Verification items for this drawing (mm, ordinates from the low corner). Round coordinates to 2 decimals unless told otherwise and drop trailing zeros. Order: outer loops, then holes, each group sorted by start corner. A loop starts at its lowest first (then second) coordinate and runs counter-clockwise, first axis right, second up. Notation, with made-up numbers: (31, -6.75) - (43, -6.75) arc R29 cw to (43, 21.25) - close; hole circle Ø11 at (-14.75, -1). An arc over 180 degrees is marked (long way). Use a Markdown table: item, result. Add a question column.
(1) Thickness scan on line 1 along Z through (x, y) = (49, 15); line 2 along Z through (x, y) = (30, 8) (1 decimal); line 3 along X through (y, z) = (27.5, 47.5) (1 decimal). Record the ranges inside material, lowest first. Write a range as [from, to].
(2) Section check A-A on y = 8. Record the boundary of the cut face in (x, z), then the cut area to 3 significant figures.
(3) Gauge pin test, flat ends, axial feed: P1, Ø5, axis at x = 12, z = 57, coming from the -Y side; P2, Ø3, axis at y = 23, z = 20, coming from the +X side (1 decimal); P3, Ø6, axis at x = 13, y = 27, coming from the -Z side; P4, Ø8, axis at y = 22.5, z = 18, coming from the +X side. Record the tip position at first contact, or that the pin passes through.
(4) Mould release check, pull along X, two halves, no side actions. Record for the marked faces 1, 2 and 3: released by +X, released by -X, zero draft, split by the parting line, or undercut.
(5) Section check B-B on y = 28.5. Record the boundary of the cut face in (x, z), then the cut area to 3 significant figures.
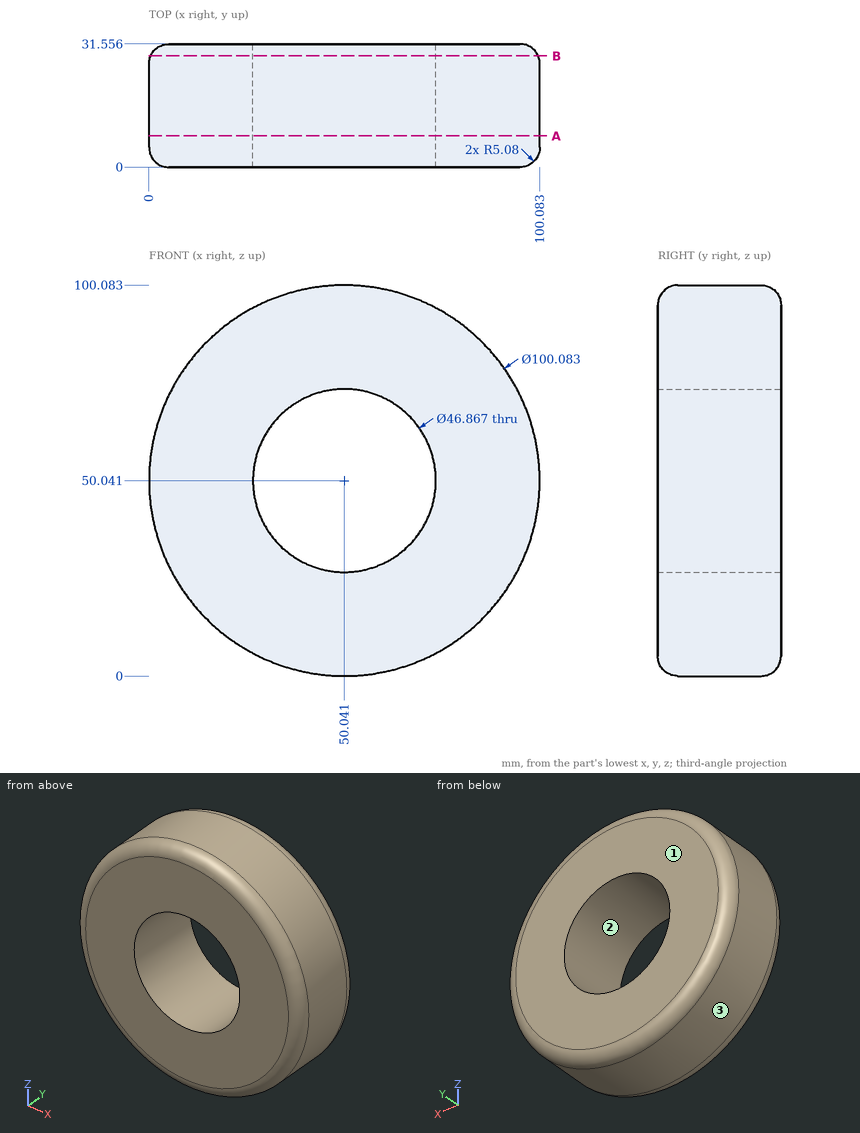
Check sheet entries:
| question | item | result |
|---|---|---|
| 1 | line 1 | z = [0.01, 26.63], [73.45, 100.07] |
| 1 | line 2 | z = [4.2, 37.9], [62.2, 95.9] |
| 1 | line 3 | x = [0.2, 26.7], [73.3, 99.9] |
| 2 | outline | circle Ø100.08 at (50.04, 50.04); hole circle Ø46.87 at (50.04, 50.04) |
| 2 | area | 6,140 mm2 |
| 3 | P1 | stops at y = 0 |
| 3 | P2 | stops at x = 91.1 |
| 3 | P3 | stops at z = 13.38 |
| 3 | P4 | stops at x = 91.49 |
| 4 | face 1 | zero draft |
| 4 | face 2 | undercut |
| 4 | face 3 | split by the parting line |
| 5 | outline | circle Ø99.24 at (50.04, 50.04); hole circle Ø46.87 at (50.04, 50.04) |
| 5 | area | 6,010 mm2 |
